```python
from build123d import *

# Parameters (mm, degrees)
F3_DEPTH  = 22.861
F5_W      = 10.16
F5_H      = 9.652
F6_DEPTH  = 0.635
F7_R      = 1.524
F8_DEPTH  = 10.16
F9_W      = 2.794
F9_H      = 6.096
F10_DEPTH = 6.6


with BuildPart() as f1:
    # F0 (on Front) → F1 (revolve)
    with BuildSketch(Plane.XZ):
        Polygon((0, 6.846469), (0, 0), (10.033, 0), (10.033, 22.86), (7.747, 22.86), (6.164025, 20.9042), (3.285246, 20.9042), (3.285246, 16.840607), (2.254922, 16.840607), (2.254922, 6.846469), (2.048858, 6.846469), align=None)
    revolve(axis=Axis((0, 0, 8.086767), (0, 0, -1)))

    # F2 (on face) → F3 (cut, through all)
    with BuildSketch(Plane(origin=(0, 0, 0), x_dir=(1, 0, 0), z_dir=(0, 0, -1))):
        with BuildLine():
            ThreePointArc((-2.1082, -1.505901), (2.5908, 0), (-2.1082, 1.505901))
            Line((-2.1082, 1.505901), (-2.1082, -1.505901))
        make_face()
    extrude(amount=-F3_DEPTH, mode=Mode.SUBTRACT)

    # F5 (on offset) → F6 (cut)
    with BuildSketch(Plane.YZ.offset(-10.16)):
        with Locations((0, 4.826)):
            Rectangle(F5_W, F5_H)
    extrude(amount=F6_DEPTH, mode=Mode.SUBTRACT)

    # F7 (on offset) → F8 (cut, through all)
    with BuildSketch(Plane.YZ.offset(-10.16)):
        with Locations((0, 4.7752)):
            Circle(F7_R)
    extrude(amount=F8_DEPTH, mode=Mode.SUBTRACT)

    # F9 (on face) → F10 (cut)
    with BuildSketch(Plane(origin=(0, 0, 0), x_dir=(1, 0, 0), z_dir=(0, 0, -1))):
        with Locations((-6.35, 0)):
            Rectangle(F9_W, F9_H)
    extrude(amount=-F10_DEPTH, mode=Mode.SUBTRACT)


solid = f1.part
```
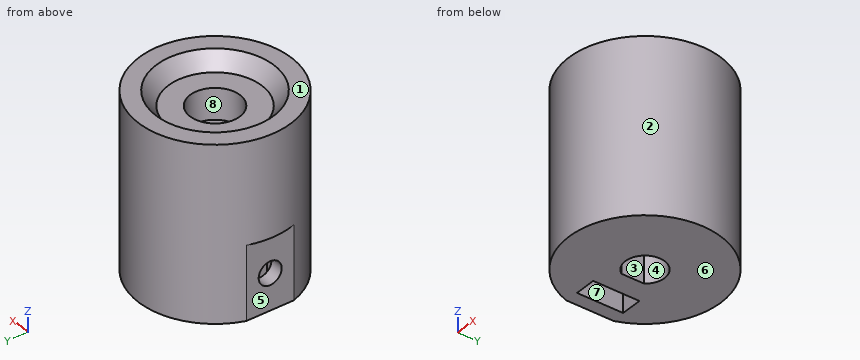
Could you check a few things on this model? Use its own coordinates, in mm. Face numbers are marked on the shaded views. A direction names the side the tool comes from. Coordinates: 2 decimals unless noted, no trailing zeros. Write each loop counter-clockwise with the first axis right and the second up, starting at its lowest first coordinate (ties: lowest second). Pieces come first, ordered by that corner, then holes. Notation, with made-up numbers: (81.5, 51.25) -> (112.5, 51.25) arc R19 ccw to (112.5, 69.25) -> close; hole circle Ø3 at (34, 55.25). An arc over 180 degrees is marked (long way). One line per question, with ' | ' between items. Start each with the question number.
1. Will these pins go through, and if not, where does the flat tip stop? P1, Ø2, axis at x = -0.5, y = 0.5, coming from the +Z side (1 decimal); P2, Ø4, axis at y = 0, z = 4.78, coming from the -X side (3 decimals); P3, Ø3.5, axis at x = 1, y = -1.5, coming from the +Z side; P4, Ø2, axis at x = -5.5, z = 4.5, coming from the +Y side.
2. For the marked faces 4, 5, 6, 7 and 8, which set-ups out of +Z, -Z, +X, -X, +Y, -Y let a thin tool reach every point of the face, with its end or its side?
3. If we section it at C-C (z = 15.75): Please give me the cut outline in (x, y), and give its area (3 significant figures).
4. Please list where these lines run through material, in increasing order: line 1 along Z through (x, y) = (-4.25, 0); line 2 along Z through (x, y) = (-8.65, 0); line 3 along X through (y, z) = (0, 9.75).
5. If we section it at D-D (z = 5.75): Please give me the cut outline in (x, y) (3 decimals), and give its area (3 significant figures).
6. If we section it at A-A (y = 0): Count the separate pieces of the cut face and the enclosed holes in it, and give its area (3 significant figures).
7. Thinking about a two-plate mould opening in Y: for the marked faces 1, 2 and 3, which applies, pulls with the +Y half, pulls with the -Y half, needs draft (parallel to the pull), parting line crosses it, or undercut?
8. If we section it at B-B (x = 0): Please give me the cut outline in (y, z).
Return value:
1) P1: passes through | P2: stops at x = -9.525 | P3: stops at z = 20.9 | P4: stops at y = 8.97
2) face 4: +Z, -Z | face 5: -Z, -X, +Y, -Y | face 6: -Z, +X, -X, +Y, -Y | face 7: -Z | face 8: +Z
3) outline: circle Ø20.07 at (0, 0); hole (-2.11, -1.51) arc R2.59 ccw (long way) to (-2.11, 1.51) -> (-2.11, 0.8) arc R2.25 ccw to (-2.11, -0.8) -> close | area: 296 mm²
4) line 1: z = 0 to 3.25, 6.3 to 20.9 | line 2: z = 0 to 3.25, 6.3 to 22.86 | line 3: x = -10.03 to -2.25, 2.59 to 10.03
5) outline: (-9.525, -3.152) arc R10.033 ccw (long way) to (-9.525, 3.152) -> (-9.525, 1.171) -> (-7.747, 1.171) -> (-7.747, 3.048) -> (-4.953, 3.048) -> (-4.953, 1.171) -> (-2.108, 1.171) -> (-2.108, 1.506) arc R2.591 cw (long way) to (-2.108, -1.506) -> (-2.108, -1.171) -> (-4.953, -1.171) -> (-4.953, -3.048) -> (-7.747, -3.048) -> (-7.747, -1.171) -> (-9.525, -1.171) -> close | area: 266 mm²
6) separate pieces: 4 | enclosed holes: 0 | area: 287 mm²
7) face 1: needs draft | face 2: parting line crosses it | face 3: undercut
8) outline: (-10.03, 0) -> (-2.59, 0) -> (-2.59, 16.84) -> (-3.29, 16.84) -> (-3.29, 20.9) -> (-6.16, 20.9) -> (-7.75, 22.86) -> (-10.03, 22.86) -> close; (2.59, 0) -> (10.03, 0) -> (10.03, 22.86) -> (7.75, 22.86) -> (6.16, 20.9) -> (3.29, 20.9) -> (3.29, 16.84) -> (2.59, 16.84) -> close
